Could you check a few things on this model? Use its own coordinates, in mm. A direction names the side the tool comes from. Coordinates: 2 decimals unless noted, no trailing zeros. Loops run counter-clockwise (first coordinate to the right, second up) from the corner with the lowest first, then second, coordinate; pieces in that order, holes last. Notation, with made-up numbers: (87, -34.5) - (96, -34.5) arc R12 cw to (96, -26.5) - close; hole circle Ø7 at (19.25, 61.5). An arc over 180 degrees is marked (long way). Use CSV: the item, a comma, the result in double quotes.
from build123d import *

# Parameters (mm, degrees)
SZKIC1_R                     = 2.55
DODANIE_WYCI_GNI_CIE11_DEPTH = 3
SZKIC7_R                     = 12.5
SZKIC7_R_2                   = 10.75
DODANIE_WYCI_GNI_CIE12_DEPTH = 2


with BuildPart() as part:
    # Szkic1 → Dodanie-wyciągnięcie11 (new body)
    with BuildSketch(Plane.XY):
        with BuildLine():
            Line((-3.026929241, 2.183576975), (22.973070759, 2.183576975))
            ThreePointArc((22.973070759, 2.183576975), (26.508604665, 0.719110881), (27.973070759, -2.816423025))
            Line((27.973070759, -2.816423025), (27.973070759, -28.816423025))
            ThreePointArc((27.973070759, -28.816423025), (26.508604665, -32.351956931), (22.973070759, -33.816423025))
            Line((22.973070759, -33.816423025), (-3.026929241, -33.816423025))
            ThreePointArc((-3.026929241, -33.816423025), (-6.562463147, -32.351956931), (-8.026929241, -28.816423025))
            Line((-8.026929241, -28.816423025), (-8.026929241, -2.816423025))
            ThreePointArc((-8.026929241, -2.816423025), (-6.562463147, 0.719110881), (-3.026929241, 2.183576975))
        make_face()
        with Locations((-2.776929241, -3.066423025)):
            Circle(SZKIC1_R, mode=Mode.SUBTRACT)
        with Locations((22.723070759, -3.066423025)):
            Circle(SZKIC1_R, mode=Mode.SUBTRACT)
        with Locations((-2.776929241, -28.566423025)):
            Circle(SZKIC1_R, mode=Mode.SUBTRACT)
        with Locations((22.723070759, -28.566423025)):
            Circle(SZKIC1_R, mode=Mode.SUBTRACT)
    extrude(amount=DODANIE_WYCI_GNI_CIE11_DEPTH)

    # Szkic7 → Dodanie-wyciągnięcie12 (add)
    with BuildSketch(Plane.XY.offset(3)):
        with Locations((9.973070759, -15.816423025)):
            Circle(SZKIC7_R)
        with Locations((9.973070759, -15.816423025)):
            Circle(SZKIC7_R_2, mode=Mode.SUBTRACT)
    extrude(amount=DODANIE_WYCI_GNI_CIE12_DEPTH)


solid = part.part
(1) Please list where these lines run through material, in increasing order: line 1 (Y direction, x = 23, z = 2.5); line 2 (Y direction, x = 21.5, z = 0.75); line 3 (Z direction, x = 26.5, y = -11).
Computed:
line 1,"y = -33.82 to -31.1, -26.03 to -5.6, -0.53 to 2.18"
line 2,"y = -33.82 to -30.8, -26.33 to -5.3, -0.83 to 2.18"
line 3,"z = 0 to 3"
(2) Suppose I cut it at C-C (z = 2). Write out the boundary of the cut face in (x, y), plus the area to 3 significant figures.
Computed:
outline,"(-8.03, -28.82) arc R5 ccw to (-3.03, -33.82) - (22.97, -33.82) arc R5 ccw to (27.97, -28.82) - (27.97, -2.82) arc R5 ccw to (22.97, 2.18) - (-3.03, 2.18) arc R5 ccw to (-8.03, -2.82) - close; hole circle Ø5.1 at (-2.78, -28.57); hole circle Ø5.1 at (-2.78, -3.07); hole circle Ø5.1 at (22.72, -28.57); hole circle Ø5.1 at (22.72, -3.07)"
area,"1,190 mm²"
(3) Suppose I cut it at A-A (x = 21.5). Write out the boundary of the cut face in (y, z), plus the area to 3 significant figures.
Computed:
outline,"(-33.82, 0) - (-30.8, 0) - (-30.8, 3) - (-33.82, 3) - close; (-26.33, 0) - (-5.3, 0) - (-5.3, 3) - (-10.98, 3) - (-10.98, 5) - (-20.65, 5) - (-20.65, 3) - (-26.33, 3) - close; (-0.83, 0) - (2.18, 0) - (2.18, 3) - (-0.83, 3) - close"
area,"100 mm²"
(4) Which directions (+Z, -Z, +X, -X, +Y, -Y) give clear straight access to the entire face, cutting with the end or side of a thin tool? Please do faces 1 (the face through (0.76, -7.37, 3.99)), 2 (the face through (-6.6, 0.68, 1.48)).
Computed:
face 1,"+Z"
face 2,"+Z, -Z, -X, +Y"
(5) Suppose I cut it at B-B (y = -14). Write out the boundary of the cut face in (x, z), plus the area to 3 significant figures.
Computed:
outline,"(-8.03, 0) - (27.97, 0) - (27.97, 3) - (22.34, 3) - (22.34, 5) - (20.57, 5) - (20.57, 3) - (-0.62, 3) - (-0.62, 5) - (-2.39, 5) - (-2.39, 3) - (-8.03, 3) - close"
area,"115 mm²"
(6) Suppose I cut it at D-D (x = 2.5). Write out the boundary of the cut face in (y, z), plus the area to 3 significant figures.
Computed:
outline,"(-33.82, 0) - (2.18, 0) - (2.18, 3) - (-5.8, 3) - (-5.8, 5) - (-8.09, 5) - (-8.09, 3) - (-23.54, 3) - (-23.54, 5) - (-25.84, 5) - (-25.84, 3) - (-33.82, 3) - close"
area,"117 mm²"
(7) Will these pins go through, and if not, where does the flat tip stop? pin 1 (8 mm diameter, centred on x = 22.72, y = -3.07, fed in from +Z); pin 2 (4.5 mm diameter, centred on x = -2.78, y = -28.57, fed in from -Z).
Computed:
pin 1,"stops at z = 3"
pin 2,"passes through"
